from build123d import *

# Parameters (mm, degrees)
EXTRUDE_1_DEPTH = 20
EXTRUDE_2_DEPTH = 9
SKETCH_4_R      = 2.9
EXTRUDE_3_DEPTH = 18


with BuildPart() as part:
    # Эскиз2 → Бобышка-Вытянуть1 (new body)
    with BuildSketch(Plane(origin=(0, 0, 0), x_dir=(1, 0, 0), z_dir=(0, 1, 0))):
        Polygon((-30.778265169, -2.685665469), (-4.786347208, -2.685665469), (-4.786347208, 58.028620245), (40.213652792, 58.028620245), (40.213652792, -56.971379755), (-39.786347208, -56.971379755), (-39.786347208, -2.685665469), align=None)
        Polygon((-34.786347208, -46.971379755), (30.213652792, -46.971379755), (30.213652792, -6.971379755), (30.213652792, 53.028620245), (5.213652792, 53.028620245), (5.213652792, -12.685665469), (-34.786347208, -12.685665469), align=None, mode=Mode.SUBTRACT)
    extrude(amount=-EXTRUDE_1_DEPTH)

    # Эскиз3 → Бобышка-Вытянуть2 (add)
    with BuildSketch(Plane(origin=(0, 0, 0), x_dir=(1, 0, 0), z_dir=(0, 1, 0))):
        Polygon((5.213652792, 53.028620245), (30.213652792, 53.028620245), (30.213652792, -46.971379755), (-34.786347208, -46.971379755), (-34.786347208, -12.685665469), (5.213652792, -12.685665469), align=None)
    extrude(amount=-EXTRUDE_2_DEPTH)

    # Эскиз4 → Бобышка-Вытянуть3 (add)
    with BuildSketch(Plane.XZ.offset(20)):
        with Locations(Location((35.213652792, 24.971379755, 0), (0, 0, 90))):
            Circle(SKETCH_4_R)
        with Locations(Location((35.213652792, 2.971379755, 0), (0, 0, 90))):
            Circle(SKETCH_4_R)
        with Locations(Location((35.213652792, -18.028620245, 0), (0, 0, 90))):
            Circle(SKETCH_4_R)
        with Locations(Location((35.213652792, -34.028620245, 0), (0, 0, 90))):
            Circle(SKETCH_4_R)
        with Locations(Location((35.213652792, -50.028620245, 0), (0, 0, 90))):
            Circle(SKETCH_4_R)
        with Locations(Location((23.213652792, 51.971379755, 0), (0, 0, 90))):
            Circle(SKETCH_4_R)
        with Locations(Location((5.213652792, 51.971379755, 0), (0, 0, 90))):
            Circle(SKETCH_4_R)
        with Locations(Location((-12.786347208, 51.971379755, 0), (0, 0, 90))):
            Circle(SKETCH_4_R)
        with Locations(Location((-30.786347208, 51.971379755, 0), (0, 0, 90))):
            Circle(SKETCH_4_R)
        with Locations(Location((-28.786347208, 7.685665469, 0), (0, 0, 90))):
            Circle(SKETCH_4_R)
        with Locations(Location((-12.786347208, 7.685665469, 0), (0, 0, 90))):
            Circle(SKETCH_4_R)
        with Locations(Location((0.213652792, -52.314334531, 0), (0, 0, 90))):
            Circle(SKETCH_4_R)
        with Locations(Location((0.213652792, -34.314334531, 0), (0, 0, 90))):
            Circle(SKETCH_4_R)
        with Locations(Location((0.213652792, -16.314334531, 0), (0, 0, 90))):
            Circle(SKETCH_4_R)
        with Locations(Location((35.213652792, 44.971379755, 0), (0, 0, 90))):
            Circle(SKETCH_4_R)
        with Locations(Location((0.213652792, 7.685665469, 0), (0, 0, 90))):
            Circle(SKETCH_4_R)
    extrude(amount=EXTRUDE_3_DEPTH)


solid = part.part
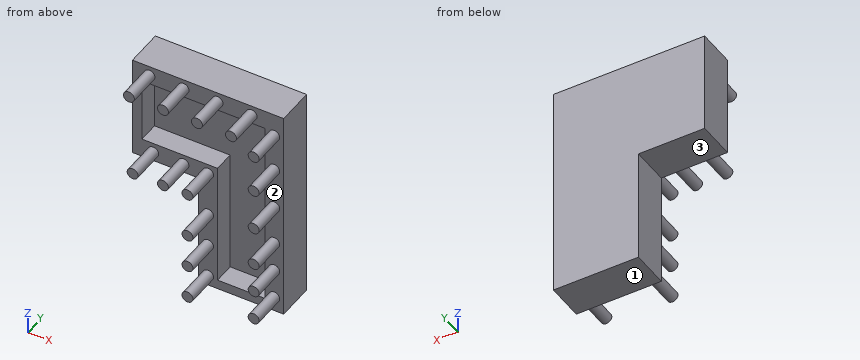
Can you work these out from the model? Positions are in its coordinate system, mm. Face numbers are marked on the shaded views. A direction names the side the tool comes from. Round coordinates to 2 decimals unless told otherwise and drop trailing zeros. Order: outer loops, then holes, each group sorted by start corner. A loop starts at its lowest first (then second) coordinate and runs counter-clockwise, first axis right, second up. Notation, with made-up numbers: (-4, -21) - (33, -21) arc R17 ccw to (33, -3) - close; hole circle Ø6 at (15.5, 39). An arc over 180 degrees is marked (long way). Answer in a Markdown table with one row per item.
(1) Which directions (+Z, -Z, +X, -X, +Y, -Y) give clear straight access to the entire face, cutting with the end or side of a thin tool? Please do the marked faces 1, 2 and 3.
From the geometry:
| item | result |
|---|---|
| face 1 | -Z, +X, -X, +Y, -Y |
| face 2 | -Y |
| face 3 | -Z, -X, +Y, -Y |
(2) Suppose I cut it at C-C, the plane z = 18. Please give me the cut outline in (x, y), plus the area to 3 significant figures.
From the geometry:
| item | result |
|---|---|
| outline | (-39.79, -20) - (-34.79, -20) - (-34.79, -9) - (30.21, -9) - (30.21, -20) - (40.21, -20) - (40.21, 0) - (-39.79, 0) - close |
| area | 885 mm2 |
(3) Suppose I cut it at D-D, the plane y = -26. Count the separate pieces of the cut face and the enclosed holes in it, plus the area to 3 significant figures.
From the geometry:
| item | result |
|---|---|
| separate pieces | 16 |
| enclosed holes | 0 |
| area | 423 mm2 |
(4) For P1, Ø16, axis at y = -7, z = -31, coming from the -X side; P2, Ø5, axis at x = 8, y = -26, coming from the -Z side; P3, Ø24, axis at x = 15, z = -15.5, coming from the -Y side; P4, Ø6, axis at x = -30, y = -9, coming from the -Z side, each with a flat end and sliding along its axis, tell me the tip position at first contact or that it passes through.
From the geometry:
| item | result |
|---|---|
| P1 | stops at x = -4.79 |
| P2 | stops at z = 49.09 |
| P3 | stops at y = -38 |
| P4 | stops at z = 2.69 |
(5) Please list where these lines run through material, in increasing order: L1, parallel to Z at x = 2, y = -13; L2, parallel to Z at x = -16.5, y = -13; L3, parallel to X at y = -12.5, z = -51.5. Write a range as from..to.
From the geometry:
| item | result |
|---|---|
| L1 | z = -58.03..12.69, 46.97..56.97 |
| L2 | z = 2.69..12.69, 46.97..56.97 |
| L3 | x = -4.79..5.21, 30.21..40.21 |
(6) Suppose I cut it at A-A, the plane y = -13. Please give me the cut outline in (x, z).
From the geometry:
| item | result |
|---|---|
| outline | (-39.79, 2.69) - (-4.79, 2.69) - (-4.79, -58.03) - (40.21, -58.03) - (40.21, 56.97) - (-39.79, 56.97) - close; hole (-34.79, 12.69) - (5.21, 12.69) - (5.21, -53.03) - (30.21, -53.03) - (30.21, 46.97) - (-34.79, 46.97) - close |
(7) Suppose I cut it at B-B, the plane x = -24. Please give me the cut outline in (y, z), plus the area to 3 significant figures.
From the geometry:
| item | result |
|---|---|
| outline | (-20, 2.69) - (0, 2.69) - (0, 56.97) - (-20, 56.97) - (-20, 46.97) - (-9, 46.97) - (-9, 12.69) - (-20, 12.69) - close |
| area | 709 mm2 |
